Source: CAD feature listing. Evaluate the final solid. Frame: model axes, mm. A direction names the side the tool comes from. Give positions to 0.01 mm unless a question says otherwise; leave off trailing zeros. Order: outer loops, then holes, each group sorted by start corner. A loop starts at its lowest first (then second) coordinate and runs counter-clockwise, first axis right, second up. Notation, with made-up numbers: M -29.5,58.5 L 2.5,58.5 A15 ccw 2.5,74.5 Z; hole C 41,77 d9. An arc over 180 degrees is marked long. Return JSON: item names as keys, results as strings.
from build123d import *

# Parameters (mm, degrees)
CYLINDER101_R               = 1.1
CYLINDER101_DEPTH           = 5
BOX013_W                    = 2
BOX013_H                    = 5.5
BOX013_DEPTH                = 5
BOX012_W                    = 0.75
BOX012_H                    = 8
BOX012_DEPTH                = 5
CYLINDER100_R               = 3
CYLINDER100_DEPTH           = 5
CUT064_PLACEMENT_ANGLE      = 120
CYLINDER104_R               = 1.1
CYLINDER104_DEPTH           = 5
CUT067_PLACEMENT_ANGLE      = -60
CYLINDER102_R               = 1.1
CYLINDER102_DEPTH           = 5
CUT065_PLACEMENT_ANGLE      = 180
CYLINDER106_R               = 1.1
CYLINDER106_DEPTH           = 5
CYLINDER103_R               = 1.1
CYLINDER103_DEPTH           = 5
CUT066_PLACEMENT_ANGLE      = 240
CYLINDER098_R               = 1.1
CYLINDER098_DEPTH           = 5
CUT063_PLACEMENT_ANGLE      = 60
CYLINDER007_R               = 19.25
CYLINDER007_DEPTH           = 5
CYLINDER018_R               = 22.5
CYLINDER018_DEPTH           = 0.5
CYLINDER070_R               = 20
CYLINDER070_DEPTH           = 5
CYLINDER006_R               = 18.5
CYLINDER006_DEPTH           = 20
CYLINDER002_R               = 22.1
CYLINDER002_DEPTH           = 17
CYLINDER001_R               = 23.5
CYLINDER001_DEPTH           = 17
CYLINDER_R                  = 23.5
CYLINDER_DEPTH              = 20
CYLINDER003_R               = 22
CYLINDER003_DEPTH           = 17
CYLINDER004_R               = 23.5
CYLINDER004_DEPTH           = 10
CUT060_PLACEMENT_ANGLE      = 180
FUSION050_PLACEMENT_ANGLE   = 180
CYLINDER073_R               = 1
CYLINDER073_DEPTH           = 10
CYLINDER073_PLACEMENT_ANGLE = 120
CYLINDER075_R               = 1
CYLINDER075_DEPTH           = 10
CYLINDER075_PLACEMENT_ANGLE = 240
CYLINDER072_R               = 1
CYLINDER072_DEPTH           = 10
CYLINDER072_PLACEMENT_ANGLE = 60
CYLINDER074_R               = 1
CYLINDER074_DEPTH           = 10
CYLINDER076_R               = 1
CYLINDER076_DEPTH           = 10
CYLINDER076_PLACEMENT_ANGLE = -60
CYLINDER071_R               = 1
CYLINDER071_DEPTH           = 10
FUSION030_PLACEMENT_ANGLE   = 30


with BuildPart() as cylinder101:
    # Cylinder101 → Cylinder101 (new body)
    with BuildSketch(Plane(origin=(15.5, 0, 15), x_dir=(1, 0, 0), z_dir=(0, 0, 1))):
        Circle(CYLINDER101_R)
    extrude(amount=CYLINDER101_DEPTH)


with BuildPart() as cube013:
    # Box013 → Box013 (new body)
    with BuildSketch(Plane(origin=(16.5, -2.75, 15), x_dir=(1, 0, 0), z_dir=(0, 0, 1))):
        with Locations((1, 2.75)):
            Rectangle(BOX013_W, BOX013_H)
    extrude(amount=BOX013_DEPTH)


with BuildPart() as cube012:
    # Box012 → Box012 (new body)
    with BuildSketch(Plane(origin=(18.2, -4, 15), x_dir=(1, 0, 0), z_dir=(0, 0, 1))):
        with Locations((0.375, 4)):
            Rectangle(BOX012_W, BOX012_H)
    extrude(amount=BOX012_DEPTH)


with BuildPart() as cylinder100:
    # Cylinder100 → Cylinder100 (new body)
    with BuildSketch(Plane(origin=(15.5, 0, 15), x_dir=(1, 0, 0), z_dir=(0, 0, 1))):
        Circle(CYLINDER100_R)
    extrude(amount=CYLINDER100_DEPTH)


with BuildPart() as cut064:
    # Fusion043 base: copy of Cylinder100
    add(cylinder100.part)

    # Fusion043: union Cube013, Cube012
    add(cube013.part)
    add(cube012.part)

    # Cut064: cut Cylinder101
    add(cylinder101.part, mode=Mode.SUBTRACT)


with BuildPart() as cut064_1:
    # Cut064 placement: moved
    add(cut064.part.moved(Location((0, 0, 9))).rotate(Axis((0, 0, 9), (0, 0, 1)), CUT064_PLACEMENT_ANGLE))


with BuildPart() as cylinder104:
    # Cylinder104 → Cylinder104 (new body)
    with BuildSketch(Plane(origin=(15.5, 0, 15), x_dir=(1, 0, 0), z_dir=(0, 0, 1))):
        Circle(CYLINDER104_R)
    extrude(amount=CYLINDER104_DEPTH)


with BuildPart() as cut067:
    # Fusion046 base: copy of Cylinder100
    add(cylinder100.part)

    # Fusion046: union Cube013, Cube012
    add(cube013.part)
    add(cube012.part)

    # Cut067: cut Cylinder104
    add(cylinder104.part, mode=Mode.SUBTRACT)


with BuildPart() as cut067_1:
    # Cut067 placement: moved
    add(cut067.part.moved(Location((0, 0, 9))).rotate(Axis((0, 0, 9), (0, 0, 1)), CUT067_PLACEMENT_ANGLE))


with BuildPart() as cylinder102:
    # Cylinder102 → Cylinder102 (new body)
    with BuildSketch(Plane(origin=(15.5, 0, 15), x_dir=(1, 0, 0), z_dir=(0, 0, 1))):
        Circle(CYLINDER102_R)
    extrude(amount=CYLINDER102_DEPTH)


with BuildPart() as cut065:
    # Fusion044 base: copy of Cylinder100
    add(cylinder100.part)

    # Fusion044: union Cube013, Cube012
    add(cube013.part)
    add(cube012.part)

    # Cut065: cut Cylinder102
    add(cylinder102.part, mode=Mode.SUBTRACT)


with BuildPart() as cut065_1:
    # Cut065 placement: moved
    add(cut065.part.moved(Location((0, 0, 9))).rotate(Axis((0, 0, 9), (0, 0, 1)), CUT065_PLACEMENT_ANGLE))


with BuildPart() as cylinder106:
    # Cylinder106 → Cylinder106 (new body)
    with BuildSketch(Plane(origin=(15.5, 0, 15), x_dir=(1, 0, 0), z_dir=(0, 0, 1))):
        Circle(CYLINDER106_R)
    extrude(amount=CYLINDER106_DEPTH)


with BuildPart() as cut069:
    # Fusion048 base: copy of Cylinder100
    add(cylinder100.part)

    # Fusion048: union Cube013, Cube012
    add(cube013.part)
    add(cube012.part)

    # Cut069: cut Cylinder106
    add(cylinder106.part, mode=Mode.SUBTRACT)


with BuildPart() as cut069_1:
    # Cut069 placement: moved
    add(cut069.part.moved(Location((0, 0, 9))))


with BuildPart() as cylinder103:
    # Cylinder103 → Cylinder103 (new body)
    with BuildSketch(Plane(origin=(15.5, 0, 15), x_dir=(1, 0, 0), z_dir=(0, 0, 1))):
        Circle(CYLINDER103_R)
    extrude(amount=CYLINDER103_DEPTH)


with BuildPart() as cut066:
    # Fusion045 base: copy of Cylinder100
    add(cylinder100.part)

    # Fusion045: union Cube013, Cube012
    add(cube013.part)
    add(cube012.part)

    # Cut066: cut Cylinder103
    add(cylinder103.part, mode=Mode.SUBTRACT)


with BuildPart() as cut066_1:
    # Cut066 placement: moved
    add(cut066.part.moved(Location((0, 0, 9))).rotate(Axis((0, 0, 9), (0, 0, 1)), CUT066_PLACEMENT_ANGLE))


with BuildPart() as cylinder098:
    # Cylinder098 → Cylinder098 (new body)
    with BuildSketch(Plane(origin=(15.5, 0, 15), x_dir=(1, 0, 0), z_dir=(0, 0, 1))):
        Circle(CYLINDER098_R)
    extrude(amount=CYLINDER098_DEPTH)


with BuildPart() as fusion049:
    # Fusion042 base: copy of Cylinder100
    add(cylinder100.part)

    # Fusion042: union Cube013, Cube012
    add(cube013.part)
    add(cube012.part)

    # Cut063: cut Cylinder098
    add(cylinder098.part, mode=Mode.SUBTRACT)


with BuildPart() as fusion049_1:
    # Cut063 placement: moved
    add(fusion049.part.moved(Location((0, 0, 9))).rotate(Axis((0, 0, 9), (0, 0, 1)), CUT063_PLACEMENT_ANGLE))

    # Fusion049: union Cut064, Cut067, Cut065, Cut069, Cut066
    add(cut064_1.part)
    add(cut067_1.part)
    add(cut065_1.part)
    add(cut069_1.part)
    add(cut066_1.part)


with BuildPart() as cylinder007:
    # Cylinder007 → Cylinder007 (new body)
    with BuildSketch(Plane.XY.offset(5)):
        Circle(CYLINDER007_R)
    extrude(amount=CYLINDER007_DEPTH)


with BuildPart() as cone:
    # Cone → Cone (revolve)
    with BuildSketch(Plane(origin=(0, 0, 5), x_dir=(1, 0, 0), z_dir=(0, -1, 0))):
        Polygon((0, 0), (20, 0), (12, 6), (0, 6), align=None)
    revolve(axis=Axis((0, 0, 5), (0, 0, 1)))


with BuildPart() as cylinder018:
    # Cylinder018 → Cylinder018 (new body)
    with BuildSketch(Plane.XY):
        Circle(CYLINDER018_R)
    extrude(amount=CYLINDER018_DEPTH)


with BuildPart() as cylinder070:
    # Cylinder070 → Cylinder070 (new body)
    with BuildSketch(Plane.XY):
        Circle(CYLINDER070_R)
    extrude(amount=CYLINDER070_DEPTH)


with BuildPart() as cylinder006:
    # Cylinder006 → Cylinder006 (new body)
    with BuildSketch(Plane.XY):
        Circle(CYLINDER006_R)
    extrude(amount=CYLINDER006_DEPTH)


with BuildPart() as cylinder002:
    # Cylinder002 → Cylinder002 (new body)
    with BuildSketch(Plane.XY):
        Circle(CYLINDER002_R)
    extrude(amount=CYLINDER002_DEPTH)


with BuildPart() as cut:
    # Cylinder001 → Cylinder001 (new body)
    with BuildSketch(Plane.XY):
        Circle(CYLINDER001_R)
    extrude(amount=CYLINDER001_DEPTH)

    # Cut: cut Cylinder002
    add(cylinder002.part, mode=Mode.SUBTRACT)


with BuildPart() as cut_1:
    # Cut placement: moved
    add(cut.part.moved(Location((0, 0, 1.5))))


with BuildPart() as cut001:
    # Cylinder → Cylinder (new body)
    with BuildSketch(Plane.XY):
        Circle(CYLINDER_R)
    extrude(amount=CYLINDER_DEPTH)

    # Cut001: cut Cut
    add(cut_1.part, mode=Mode.SUBTRACT)


with BuildPart() as cylinder003:
    # Cylinder003 → Cylinder003 (new body)
    with BuildSketch(Plane.XY):
        Circle(CYLINDER003_R)
    extrude(amount=CYLINDER003_DEPTH)


with BuildPart() as rim_inner_rear:
    # Cylinder004 → Cylinder004 (new body)
    with BuildSketch(Plane.XY.offset(0.5)):
        Circle(CYLINDER004_R)
    extrude(amount=CYLINDER004_DEPTH)

    # Cut002: cut Cylinder003
    add(cylinder003.part, mode=Mode.SUBTRACT)


with BuildPart() as rim_inner_rear_1:
    # Cut002 placement: moved
    add(rim_inner_rear.part.moved(Location((0, 0, 4.5))))

    # Fusion: union Cut001
    add(cut001.part)

    # Cut031: cut Cylinder006
    add(cylinder006.part, mode=Mode.SUBTRACT)

    # Cut057: cut Cylinder070
    add(cylinder070.part, mode=Mode.SUBTRACT)

    # Cut058: cut Cylinder018
    add(cylinder018.part, mode=Mode.SUBTRACT)

    # Cut059: cut Cone
    add(cone.part, mode=Mode.SUBTRACT)

    # Cut060: cut Cylinder007
    add(cylinder007.part, mode=Mode.SUBTRACT)


with BuildPart() as rim_inner_rear_2:
    # Cut060 placement: moved
    add(rim_inner_rear_1.part.moved(Location((0, 0, 44))).rotate(Axis((0, 0, 44), (0, 1, 0)), CUT060_PLACEMENT_ANGLE))

    # Fusion050: union Fusion049
    add(fusion049_1.part)


with BuildPart() as rim_inner_rear_3:
    # Fusion050 placement: moved
    add(rim_inner_rear_2.part.rotate(Axis((0, 0, 0), (0, 1, 0)), FUSION050_PLACEMENT_ANGLE))


with BuildPart() as cylinder073:
    # Cylinder073 → Cylinder073 (new body)
    with BuildSketch(Plane.XY):
        Circle(CYLINDER073_R)
    extrude(amount=CYLINDER073_DEPTH)


with BuildPart() as cylinder073_1:
    # Cylinder073 placement: moved
    add(cylinder073.part.moved(Location((-9.25, 16.02147, 5))).rotate(Axis((-9.25, 16.02147, 5), (0, 0, 1)), CYLINDER073_PLACEMENT_ANGLE))


with BuildPart() as cylinder075:
    # Cylinder075 → Cylinder075 (new body)
    with BuildSketch(Plane.XY):
        Circle(CYLINDER075_R)
    extrude(amount=CYLINDER075_DEPTH)


with BuildPart() as cylinder075_1:
    # Cylinder075 placement: moved
    add(cylinder075.part.moved(Location((-9.25, -16.02147, 5))).rotate(Axis((-9.25, -16.02147, 5), (0, 0, 1)), CYLINDER075_PLACEMENT_ANGLE))


with BuildPart() as cylinder072:
    # Cylinder072 → Cylinder072 (new body)
    with BuildSketch(Plane.XY):
        Circle(CYLINDER072_R)
    extrude(amount=CYLINDER072_DEPTH)


with BuildPart() as cylinder072_1:
    # Cylinder072 placement: moved
    add(cylinder072.part.moved(Location((9.25, 16.02147, 5))).rotate(Axis((9.25, 16.02147, 5), (0, 0, 1)), CYLINDER072_PLACEMENT_ANGLE))


with BuildPart() as cylinder074:
    # Cylinder074 → Cylinder074 (new body)
    with BuildSketch(Plane(origin=(-18.5, 0, 5), x_dir=(-1, 0, 0), z_dir=(0, 0, 1))):
        Circle(CYLINDER074_R)
    extrude(amount=CYLINDER074_DEPTH)


with BuildPart() as cylinder076:
    # Cylinder076 → Cylinder076 (new body)
    with BuildSketch(Plane.XY):
        Circle(CYLINDER076_R)
    extrude(amount=CYLINDER076_DEPTH)


with BuildPart() as cylinder076_1:
    # Cylinder076 placement: moved
    add(cylinder076.part.moved(Location((9.25, -16.02147, 5))).rotate(Axis((9.25, -16.02147, 5), (0, 0, 1)), CYLINDER076_PLACEMENT_ANGLE))


with BuildPart() as fusion070:
    # Cylinder071 → Cylinder071 (new body)
    with BuildSketch(Plane(origin=(18.5, 0, 5), x_dir=(1, 0, 0), z_dir=(0, 0, 1))):
        Circle(CYLINDER071_R)
    extrude(amount=CYLINDER071_DEPTH)

    # Fusion030: union Cylinder073, Cylinder075, Cylinder072, Cylinder074, Cylinder076
    add(cylinder073_1.part)
    add(cylinder075_1.part)
    add(cylinder072_1.part)
    add(cylinder074.part)
    add(cylinder076_1.part)


with BuildPart() as fusion070_1:
    # Fusion030 placement: moved
    add(fusion070.part.moved(Location((0, 0, -39))).rotate(Axis((0, 0, -39), (0, 0, 1)), FUSION030_PLACEMENT_ANGLE))

    # Fusion070: union rim-inner-rear_
    add(rim_inner_rear_3.part)


solid = fusion070_1.part
1. Draft query along Y for faces 1 (the face through (15.166, -8.731, -29.07)), 2 (the face through (-14.4, 0, -26.5)), 3 (the face through (0, -23, -44)). Return one class per face: pulls with the +Y half, pulls with the -Y half, needs draft (parallel to the pull), parting line crosses it, or undercut.
Evaluation:
{"face 1": "undercut", "face 2": "undercut", "face 3": "needs draft"}
2. Ray query, probe 1 along Z at (x, y) = (-9.5, -21); probe 2 along Z at (x, y) = (-9.5, -20); probe 3 along Y at (x, z) = (-7.75, -27.35). Return the intervals inside material, ascending.
Evaluation:
{"probe 1": "z = -44 to -42.5, -39 to -29, -25.5 to -24", "probe 2": "z = -43.5 to -42.5, -39 to -29, -25.5 to -24", "probe 3": "y = -20.7 to -14.52, -12.32 to -10.42, 10.42 to 12.32, 14.52 to 20.7"}
3. Section query A-A (z = -41.5). Return loops of the section in (x, y).
Evaluation:
{"outline": "C 0,0 d44.2; hole C 0,0 d40"}
4. Set-up query: faces 4 (the face through (8, 15, -29)), 5 (the face through (-17, 2.75, -26)), 6 (the face through (16, 16, -29)). Return all of +Z, -Z, +X, -X, +Y, -Y with unobstructed straight access to the full face (end or side cutting, diameter ignored); none if empty.
Evaluation:
{"face 4": "-Z", "face 5": "+Z, -Z", "face 6": "none"}
5. Section query B-B (x = -21). Return loops of the section in (y, z).
Evaluation:
{"outline": "M -10.55,-44 L -8.08,-44 L -8.08,-43.5 L 8.08,-43.5 L 8.08,-44 L 10.55,-44 L 10.55,-42.5 L 6.89,-42.5 L 6.89,-39 L 10.55,-39 L 10.55,-29 L 6.89,-29 L 6.89,-25.5 L 10.55,-25.5 L 10.55,-24 L -10.55,-24 L -10.55,-25.5 L -6.89,-25.5 L -6.89,-29 L -10.55,-29 L -10.55,-39 L -6.89,-39 L -6.89,-42.5 L -10.55,-42.5 Z"}
6. First-contact query: pin 1 (14 mm diameter, centred on x = -6, y = 10, fed in from -Z); pin 2 (6 mm diameter, centred on x = 10.5, z = -28, fed in from -Y); pin 3 (12 mm diameter, centred on x = -2, z = -28.5, fed in from -Y). Flat tips, straight axial feed; report the tip coordinate or a pass-through.
Evaluation:
{"pin 1": "stops at z = -34", "pin 2": "stops at y = -22.21", "pin 3": "stops at y = -23.5"}
